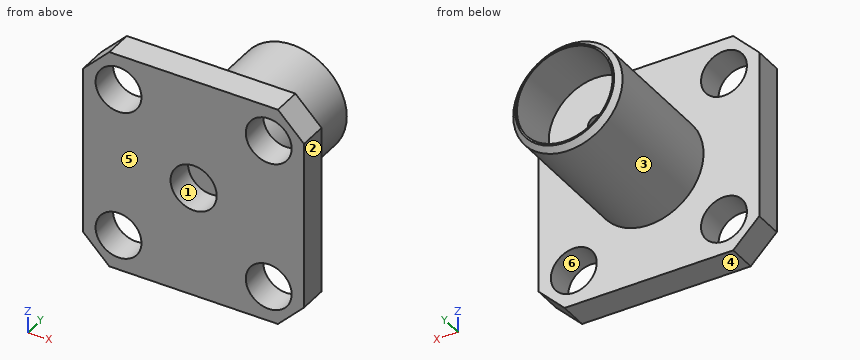
Autodesk Inventor part; units mm, degrees
ref_plane "YZ Plane" through (0, 0, 0) normal (1, 0, 0) x (0, 1, 0)
ref_plane "XZ Plane" through (0, 0, 0) normal (0, 1, 0) x (-1, 0, 0)
ref_plane "XY Plane" through (0, 0, 0) normal (0, 0, 1) x (1, 0, 0)
sketch "Sketch1" plane through (0, 0, 0) normal (0, 1, 0) x (-1, 0, 0)
  line L0 (4.85, 6.35) -> (-4.85, 6.35)
  line L1 (-6.35, 4.85) -> (-6.35, -4.85)
  line L2 (-4.85, -6.35) -> (4.85, -6.35)
  line L3 (6.35, -4.85) -> (6.35, 4.85)
  line L4 (6.35, 6.35) -> (-6.35, -6.35) construction
  line L5 (-6.35, 6.35) -> (6.35, -6.35) construction
  line L6 (6.35, -4.85) -> (4.85, -6.35)
  line L7 (-4.85, -6.35) -> (-6.35, -4.85)
  line L8 (-4.85, 6.35) -> (-6.35, 4.85)
  line L9 (6.35, 4.85) -> (4.85, 6.35)
  line L10 (4.32, 4.32) -> (-4.32, 4.32) construction
  line L11 (-4.32, 4.32) -> (-4.32, -4.32) construction
  line L12 (-4.32, -4.32) -> (4.32, -4.32) construction
  line L13 (4.32, -4.32) -> (4.32, 4.32) construction
  line L14 (4.32, 4.32) -> (-4.32, -4.32) construction
  line L15 (-4.32, 4.32) -> (4.32, -4.32) construction
  circle A0 centre (0, 0) radius 1.3272
  dimension "d0" = 12.7
  dimension "d1" = 12.7
  dimension "d5" = 9.7
  dimension "d6" = 1.5
  dimension "d7" = 8.64
  dimension "d8" = 8.64
  dimension "d9" = 2.6543
extrude "Extrusion1" add sketch "Sketch1" along normal blind 1.65
sketch "Sketch2" plane through (0, 1.65, 0) normal (0, 1, 0) x (1, 0, 0)
  circle A0 centre (0, 0) radius 1.3272
  line L0 (-4.32, -4.32) -> (4.32, -4.32) construction
  line L1 (4.32, -4.32) -> (4.32, 4.32) construction
  line L2 (4.32, 4.32) -> (-4.32, 4.32) construction
  line L3 (-4.32, 4.32) -> (-4.32, -4.32) construction
  line L4 (-4.32, -4.32) -> (4.32, 4.32) construction
  line L5 (4.32, -4.32) -> (-4.32, 4.32) construction
  dimension "d12" = 8.64
  dimension "d13" = 8.64
hole "Hole1" at (-4.32, 1.65, -4.32) at (4.32, 1.65, -4.32) at (4.32, 1.65, 4.32) at (-4.32, 1.65, 4.32) direction (0, -1, 0) diameter 2.64 depth 1.65 tip angle 118
sketch "Sketch3" plane through (0, 1.65, 0) normal (0, 1, 0) x (1, 0, 0)
  circle A0 centre (0, 0) radius 1.3272
  circle A1 centre (0, 0) radius 3.145
  dimension "d21" = 6.29
extrude "Extrusion2" add sketch "Sketch3" along normal blind 7.93 contours A0 | A1
thread "Thread1"
chamfer "Chamfer1" distance 0.3 angle 45 1 edges at (-3.145, 9.58, 0)
sketch "Sketch4" plane through (0, 9.58, 0) normal (0, 1, 0) x (1, 0, 0)
  circle A0 centre (0, 0) radius 2.845
  circle A1 centre (0, 0) radius 2.75
  dimension "d30" = 5.5
extrude "Extrusion3" cut sketch "Sketch4" against normal blind 3 contours A1
sketch "Sketch5" plane through (0, 1.65, 0) normal (0, -1, 0) x (1, 0, 0)
  circle A0 centre (0, 0) radius 1.3272
  circle A1 centre (0, 0) radius 0.254
  dimension "d33" = 0.508
extrude "Extrusion4" cut sketch "Sketch5" against normal blind 6 contours A1
sketch "Sketch6" plane through (0, 6.58, 0) normal (0, 1, 0) x (1, 0, 0)
  circle A0 centre (0, 0) radius 0.254
  circle A1 centre (0, 0) radius 2.75
  circle A2 centre (0, 0) radius 0.5
  dimension "d36" = 1
extrude "Extrusion5" cut sketch "Sketch6" against normal blind 2 contours A2
properties part number "SMA_connector"
Model file for the job. Use its own axes, mm. Face numbers are marked on the shaded views. A direction names the side the tool comes from. Coordinates: 2 decimals unless noted, no trailing zeros. Loops run counter-clockwise (first coordinate to the right, second up) from the corner with the lowest first, then second, coordinate; pieces in that order, holes last. Notation, with made-up numbers: (-25, 84.5) -> (16, 84.5) arc R7 ccw to (16, 89.5) -> close; hole circle Ø8 at (-24.75, 16.25). An arc over 180 degrees is marked (long way). Answer as a JSON object with one key per item and string values.
Q1. Cut at D-D (x = -4.32). List the corners of the cut face in (y, z).
Report:
{"outline": "(0, -6.35) -> (1.65, -6.35) -> (1.65, -5.64) -> (0, -5.64) -> close; (0, -3) -> (1.65, -3) -> (1.65, 3) -> (0, 3) -> close; (0, 5.64) -> (1.65, 5.64) -> (1.65, 6.35) -> (0, 6.35) -> close"}
Q2. Cut at C-C (z = -4.32). List the corners of the cut face in (x, y).
Report:
{"outline": "(-6.35, 0) -> (-5.64, 0) -> (-5.64, 1.65) -> (-6.35, 1.65) -> close; (-3, 0) -> (3, 0) -> (3, 1.65) -> (-3, 1.65) -> close; (5.64, 0) -> (6.35, 0) -> (6.35, 1.65) -> (5.64, 1.65) -> close"}
Q3. Cut at B-B (x = 0). List the corners of the cut face in (y, z) (3 decimals).
Report:
{"outline": "(0, -6.35) -> (1.65, -6.35) -> (1.65, -3.145) -> (9.28, -3.145) -> (9.58, -2.845) -> (9.58, -2.75) -> (6.58, -2.75) -> (6.58, -0.5) -> (4.58, -0.5) -> (4.58, -0.254) -> (1.65, -0.254) -> (1.65, -1.327) -> (0, -1.327) -> close; (0, 1.327) -> (1.65, 1.327) -> (1.65, 0.254) -> (4.58, 0.254) -> (4.58, 0.5) -> (6.58, 0.5) -> (6.58, 2.75) -> (9.58, 2.75) -> (9.58, 2.845) -> (9.28, 3.145) -> (1.65, 3.145) -> (1.65, 6.35) -> (0, 6.35) -> close"}
Q4. Pull direction Z, two halves, no side cores. Call the marked faces 4, 5 and 6: released by +Z, released by -Z, zero draft, split by the parting line, or undercut.
Report:
{"face 4": "released by -Z", "face 5": "zero draft", "face 6": "undercut"}
Q5. Probe probe 1 along Z at (x, y) = (4.32, 0.7); probe 2 along Y at (x, z) = (-1.5, -3.75). List the from-to ranges inside material, lowest first.
Report:
{"probe 1": "z = -6.35 to -5.64, -3 to 3, 5.64 to 6.35", "probe 2": "y = 0 to 1.65"}
Q6. Cut at A-A (z = 0). List the corners of the cut face in (x, y) (3 decimals), and give its area (3 significant figures).
Report:
{"outline": "(-6.35, 0) -> (-1.327, 0) -> (-1.327, 1.65) -> (-0.254, 1.65) -> (-0.254, 4.58) -> (-0.5, 4.58) -> (-0.5, 6.58) -> (-2.75, 6.58) -> (-2.75, 9.58) -> (-2.845, 9.58) -> (-3.145, 9.28) -> (-3.145, 1.65) -> (-6.35, 1.65) -> close; (0.254, 1.65) -> (1.327, 1.65) -> (1.327, 0) -> (6.35, 0) -> (6.35, 1.65) -> (3.145, 1.65) -> (3.145, 9.28) -> (2.845, 9.58) -> (2.75, 9.58) -> (2.75, 6.58) -> (0.5, 6.58) -> (0.5, 4.58) -> (0.254, 4.58) -> close", "area": "46.4 mm2"}
Q7. 3-axis set-ups, long thin cutter, end or side, ignore diameter. For the marked faces 1, 2 and 3: which of +Z, -Z, +X, -X, +Y, -Y reach the whole face in a straight line?
Report:
{"face 1": "-Y", "face 2": "+Z, -Z, +X, +Y, -Y", "face 3": "+Y"}
Q8. Flat gauge pins, fed straight in: P1, Ø6, axis at x = -0.5, z = 1, coming from the +Y side; P2, Ø4, axis at y = 4, z = -1.5, coming from the -X side (3 decimals); P3, Ø4, axis at x = 0, z = 0, coming from the +Y side; P4, Ø0.8, axis at x = 0, z = 0.5, coming from the -Y side. Where does each tip first touch, or does it go through?
Report:
{"P1": "stops at y = 9.58", "P2": "stops at x = -3.145", "P3": "stops at y = 6.58", "P4": "stops at y = 1.65"}
